from build123d import *

# Parameters (mm, degrees)
BOSS_EXTRUDE1_DEPTH     = 24.13
CUT_EXTRUDE1_DEPTH      = 140.018460965
CUT_EXTRUDE1_DEPTH_BACK = 140.018460965
SKETCH2_R               = 1.5113
SKETCH2_R_2             = 4.7625
BOSS_EXTRUDE2_DEPTH     = 3.302
CUT_EXTRUDE2_DEPTH      = 140.247845391
CUT_EXTRUDE2_DEPTH_BACK = 140.247845391
FILLET1_R               = 1.778
CUT_EXTRUDE3_DEPTH      = 0.889


with BuildPart() as part:
    # Sketch1 → Boss-Extrude1 (new body)
    with BuildSketch(Plane.XY):
        Polygon((0, 0), (-52.832, 0), (-111.252, 6.498782895), (-136.652, 8.382), (-136.407851909, 11.674961541), (-110.947287613, 9.787254053), (-52.648903452, 3.302), (0, 3.302), align=None)
    extrude(amount=BOSS_EXTRUDE1_DEPTH)

    # Sketch2 → Cut-Extrude1 (cut, two sides: drawn at the far end of the back side and taken through both)
    with BuildSketch(Plane(origin=(0, 3.302, 0), x_dir=(1, 0, 0), z_dir=(0, 1, 0)).offset(-CUT_EXTRUDE1_DEPTH_BACK)):
        with Locations(Location((-6.324451726, -12.7, 0), (0, 0, 180))):
            Circle(SKETCH2_R)
        with Locations(Location((-46.324451726, -12.7, 0), (0, 0, 180))):
            Circle(SKETCH2_R)
        with Locations(Location((-66.324451726, -12.7, 0), (0, 0, 180))):
            Circle(SKETCH2_R_2)
        with Locations(Location((-86.324451726, -12.7, 0), (0, 0, 180))):
            Circle(SKETCH2_R_2)
        with Locations(Location((-106.324451726, -12.7, 0), (0, 0, 180))):
            Circle(SKETCH2_R_2)
        with Locations(Location((-126.324451726, -12.7, 0), (0, 0, 180))):
            Circle(SKETCH2_R_2)
    extrude(amount=CUT_EXTRUDE1_DEPTH + CUT_EXTRUDE1_DEPTH_BACK, mode=Mode.SUBTRACT)

    # Sketch3 → Boss-Extrude2 (add)
    with BuildSketch(Plane(origin=(0.115129755, 1.552819246, 0), x_dir=(0.9972627319520296, -0.07393945806924965, 0), z_dir=(0.07393945806924965, 0.9972627319520296, 0))):
        with BuildLine():
            Line((-136.897707384, 0), (-136.897707384, 8.89))
            ThreePointArc((-136.897707384, 8.89), (-131.63888491, 16.361853382), (-122.830660339, 13.933070421))
            Line((-122.830660339, 13.933070421), (-111.367259408, 0))
            Line((-111.367259408, 0), (-136.897707384, 0))
        make_face()
    extrude(amount=-BOSS_EXTRUDE2_DEPTH)

    # Sketch4 → Cut-Extrude2 (cut, two sides: drawn at the far end of the back side and taken through both)
    with BuildSketch(Plane(origin=(0.115129755, 1.552819246, 0), x_dir=(0.9972627319520296, -0.07393945806924965, 0), z_dir=(0.07393945806924965, 0.9972627319520296, 0)).offset(-CUT_EXTRUDE2_DEPTH_BACK)):
        Polygon((-136.897707384, 8.89), (-134.992707384, -24.13), (-136.897707384, -24.13), (-138.802707384, -24.13), (-138.802707384, 8.89), align=None)
    extrude(amount=CUT_EXTRUDE2_DEPTH + CUT_EXTRUDE2_DEPTH_BACK, mode=Mode.SUBTRACT)

    # Fillet1
    fillet1_edges = [part.edges().sort_by_distance(p)[0] for p in [
        (0, 1.651, 0),
        (0, 1.651, 24.13),
        (-134.63014045, 9.887626103, 24.13),
    ]]
    fillet(fillet1_edges, radius=FILLET1_R)

    # Sketch5 → Cut-Extrude3 (cut)
    with BuildSketch(Plane(origin=(0.115129755, 1.552819246, 0), x_dir=(0.9972627319520296, -0.07393945806924965, 0), z_dir=(0.07393945806924965, 0.9972627319520296, 0))):
        with BuildLine():
            Line((-135.786917217, 4.840316171), (-136.644610097, 4.502980352))
            Line((-136.644610097, 4.502980352), (-136.88295075, 8.406219254))
            ThreePointArc((-136.88295075, 8.406219254), (-131.865445622, 16.27671084), (-122.830660339, 13.933070421))
            Line((-122.830660339, 13.933070421), (-120.346128436, 10.913272179))
            Line((-120.346128436, 10.913272179), (-121.203821316, 10.57593636))
            ThreePointArc((-121.203821316, 10.57593636), (-126.054969147, 1.50328916), (-135.786917217, 4.840316171))
        make_face()
    extrude(amount=-CUT_EXTRUDE3_DEPTH, mode=Mode.SUBTRACT)


solid = part.part
Geometry: final body of the model. Coordinates: model frame, mm. Give positions to 0.01 mm unless a question says otherwise; leave off trailing zeros. Write each loop counter-clockwise with the first axis right and the second up, starting at its lowest first coordinate (ties: lowest second). Pieces come first, ordered by that corner, then holes. Notation, with made-up numbers: (13.5, -21) -> (32.5, -21) arc R17 ccw to (32.5, -6) -> close; hole circle Ø9 at (18.5, 46.5). An arc over 180 degrees is marked (long way). Answer as a JSON object with one key per item and string values.
1. Cut plane B-B on x = -32. Output: boundary loops of the cut face in (y, z), and give its area (3 significant figures).
Ans:
{"outline": "(0, 0) -> (3.3, 0) -> (3.3, 24.13) -> (0, 24.13) -> close", "area": "79.7 mm^2"}
2. Mould query, pull axis Z, two halves, no side actions, for faces 1 (the cylindrical face through (-82.814, 5.331, 15.919)), 2 (the flat face through (-56, 3, 0)), 3 (the cylindrical face through (-121.567, 9.227, 12.909)), 4 (the flat face through (-27, 3.302, 12)). Classes: pulls with the +Z half, pulls with the -Z half, needs draft (parallel to the pull), parting line crosses it, or undercut.
Ans:
{"face 1": "undercut", "face 2": "pulls with the -Z half", "face 3": "undercut", "face 4": "needs draft"}
3. Cut plane D-D on x = -58.5. Output: boundary loops of the cut face in (y, z).
Ans:
{"outline": "(0.63, 0) -> (3.95, 0) -> (3.95, 24.13) -> (0.63, 24.13) -> close"}
4. Cut plane A-A on z = 5. Output: boundary loops of the cut face in (x, y).
Ans:
{"outline": "(-135.85, 8.32) -> (-111.25, 6.5) -> (-52.83, 0) -> (0, 0) -> (0, 3.3) -> (-52.65, 3.3) -> (-110.95, 9.79) -> (-135.61, 11.62) -> close"}
5. Contact query for flat-ended pins moving along their axis: pin 1 (5 mm diameter, centred on x = -14, y = 5, fed in from -Z); pin 2 (12 mm diameter, centred on x = -37, z = 15, fed in from +Y); pin 3 (6 mm diameter, centred on x = -37.5, y = 8, fed in from -Z); pin 4 (11 mm diameter, centred on x = -126.32, z = 12.7, fed in from +Y). Output: stop coordinate, or through.
Ans:
{"pin 1": "stops at z = 0", "pin 2": "stops at y = 3.3", "pin 3": "passes through", "pin 4": "stops at y = 11.33"}
6. Cut plane C-C on z = 21. Output: boundary loops of the cut face in (x, y).
Ans:
{"outline": "(-134.93, 8.25) -> (-111.25, 6.5) -> (-52.83, 0) -> (0, 0) -> (0, 3.3) -> (-52.65, 3.3) -> (-110.95, 9.79) -> (-134.69, 11.55) -> close"}
7. Ray query, probe 1 along Z at (x, y) = (-106, 7.5); probe 2 along Z at (x, y) = (-47.5, 2.25); probe 3 along Y at (x, z) = (-7, 10.5). Return the intervals inside material, ascending. Write a range as from..to.
Ans:
{"probe 1": "z = 0..7.95, 17.45..24.13", "probe 2": "z = 0..11.75, 13.65..24.13", "probe 3": "y = 0..3.3"}
